```python
from build123d import *

# Parameters (mm, degrees)
SKETCH1_W                    = 152.4
SKETCH1_H                    = 6.35
BOSS_EXTRUDE1_DEPTH          = 126.8095
F_3_4_0_75_DIAMETER_HOLE1_D  = 19.05
CUT_EXTRUDE1_DEPTH           = 199.360106348
FILLET1_R                    = 3.81
FILLET4_R                    = 3.175
F_5_8_0_625_DIAMETER_HOLE1_D = 15.875
F_10_24_TAPPED_HOLE1_D       = 3.7973
F_10_24_TAPPED_HOLE1_DEPTH   = 19.05
F_10_24_TAPPED_HOLE1_TIP     = 1.140824014
F_10_24_TAPPED_HOLE2_D       = 3.7973
F_10_24_TAPPED_HOLE2_DEPTH   = 19.05
F_10_24_TAPPED_HOLE2_TIP     = 1.140824014


with BuildPart() as part:
    # Sketch1 → Boss-Extrude1 (new, symmetric)
    with BuildSketch(Plane.XY):
        with Locations((76.2, 3.175)):
            Rectangle(SKETCH1_W, SKETCH1_H)
    extrude(amount=BOSS_EXTRUDE1_DEPTH, both=True)

    # 3/4 (0.75) Diameter Hole1 (through all)
    with Locations(Plane(origin=(0, 6.35, 0), x_dir=(1, 0, 0), z_dir=(0, 1, 0))):
        with Locations((19.05, 0), (133.35, 0)):
            Hole(F_3_4_0_75_DIAMETER_HOLE1_D / 2)

    # Sketch4 → Cut-Extrude1 (cut, through all)
    with BuildSketch(Plane(origin=(0, 6.35, 0), x_dir=(1, 0, 0), z_dir=(0, 1, 0))):
        with BuildLine():
            Line((37.010512242, -6.35), (64.976021122, -6.35))
            Line((64.976021122, -6.35), (12.7, -93.346011817))
            Line((12.7, -93.346011817), (12.7, -17.960512242))
            ThreePointArc((12.7, -17.960512242), (27.259871939, -17.190128061), (37.010512242, -6.35))
        make_face()
        with BuildLine():
            Line((12.7, 93.346011817), (64.976021122, 6.35))
            Line((64.976021122, 6.35), (37.010512242, 6.35))
            ThreePointArc((37.010512242, 6.35), (27.259871939, 17.190128061), (12.7, 17.960512242))
            Line((12.7, 17.960512242), (12.7, 93.346011817))
        make_face()
        Polygon((137.360297537, 114.1095), (82.55, 22.896029849), (82.55, 114.1095), align=None)
        Polygon((15.039702463, 114.1095), (69.85, 22.896029849), (69.85, 114.1095), align=None)
        with BuildLine():
            Line((139.7, 93.346011817), (87.423978878, 6.35))
            Line((87.423978878, 6.35), (115.389487758, 6.35))
            ThreePointArc((115.389487758, 6.35), (125.140128061, 17.190128061), (139.7, 17.960512242))
            Line((139.7, 17.960512242), (139.7, 93.346011817))
        make_face()
        Polygon((15.039702463, -114.1095), (69.85, -114.1095), (69.85, -22.896029849), align=None)
        with BuildLine():
            Line((139.7, -93.346011817), (139.7, -17.960512242))
            ThreePointArc((139.7, -17.960512242), (125.140128061, -17.190128061), (115.389487758, -6.35))
            Line((115.389487758, -6.35), (87.423978878, -6.35))
            Line((87.423978878, -6.35), (139.7, -93.346011817))
        make_face()
        Polygon((82.55, -22.896029849), (137.360297537, -114.1095), (82.55, -114.1095), align=None)
    extrude(amount=-CUT_EXTRUDE1_DEPTH, mode=Mode.SUBTRACT)

    # Fillet1
    fillet1_edges = [part.edges().sort_by_distance(p)[0] for p in [
        (64.976021122, 3.175, 6.35),
        (12.7, 3.175, 93.346011817),
        (12.7, 3.175, 17.960512242),
        (37.010512242, 3.175, 6.35),
        (139.7, 3.175, -93.346011817),
        (139.7, 3.175, -17.960512242),
        (115.389487758, 3.175, -6.35),
        (87.423978878, 3.175, -6.35),
        (115.389487758, 3.175, 6.35),
        (139.7, 3.175, 17.960512242),
        (139.7, 3.175, 93.346011817),
        (87.423978878, 3.175, 6.35),
        (12.7, 3.175, -17.960512242),
        (12.7, 3.175, -93.346011817),
        (64.976021122, 3.175, -6.35),
        (37.010512242, 3.175, -6.35),
        (15.039702463, 3.175, 114.1095),
        (69.85, 3.175, 22.896029849),
        (69.85, 3.175, 114.1095),
        (137.360297537, 3.175, 114.1095),
        (82.55, 3.175, 114.1095),
        (82.55, 3.175, 22.896029849),
        (82.55, 3.175, -114.1095),
        (137.360297537, 3.175, -114.1095),
        (82.55, 3.175, -22.896029849),
        (15.039702463, 3.175, -114.1095),
        (69.85, 3.175, -114.1095),
        (69.85, 3.175, -22.896029849),
    ]]
    fillet(fillet1_edges, radius=FILLET1_R)

    # Fillet4
    fillet4_edges = [part.edges().sort_by_distance(p)[0] for p in [
        (142.875, 6.35, 0),
        (142.875, 0, 0),
        (28.575, 6.35, 0),
        (28.575, 0, 0),
    ]]
    fillet(fillet4_edges, radius=FILLET4_R - 0.0001)  # a hair under: the kernel refuses the full size

    # 5/8 (0.625) Diameter Hole1 (through all)
    with Locations(Plane(origin=(0, 0, 0), x_dir=(-1, 0, 0), z_dir=(0, -1, 0))):
        with Locations((-76.2, 17.4625), (-76.2, -17.4625)):
            Hole(F_5_8_0_625_DIAMETER_HOLE1_D / 2)

    # #10-24 Tapped Hole1
    with Locations(Plane.XY.offset(126.8095)):
        with Locations((127, 3.175), (25.4, 3.175)):
            Hole(F_10_24_TAPPED_HOLE1_D / 2, depth=F_10_24_TAPPED_HOLE1_DEPTH)
            with Locations((0, 0, -(F_10_24_TAPPED_HOLE1_DEPTH + F_10_24_TAPPED_HOLE1_TIP / 2))):  # 118° drill point
                Cone(0, F_10_24_TAPPED_HOLE1_D / 2, F_10_24_TAPPED_HOLE1_TIP, mode=Mode.SUBTRACT)

    # #10-24 Tapped Hole2
    with Locations(Plane(origin=(0, 0, -126.8095), x_dir=(-1, 0, 0), z_dir=(0, 0, -1))):
        with Locations((-25.4, 3.175), (-127, 3.175)):
            Hole(F_10_24_TAPPED_HOLE2_D / 2, depth=F_10_24_TAPPED_HOLE2_DEPTH)
            with Locations((0, 0, -(F_10_24_TAPPED_HOLE2_DEPTH + F_10_24_TAPPED_HOLE2_TIP / 2))):  # 118° drill point
                Cone(0, F_10_24_TAPPED_HOLE2_D / 2, F_10_24_TAPPED_HOLE2_TIP, mode=Mode.SUBTRACT)


solid = part.part
```
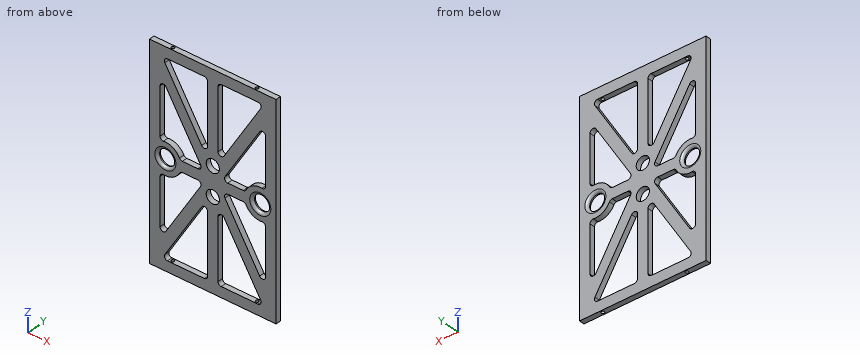
Here's how the part is built. I have some questions about the finished solid (model axes, mm). Coordinates: 2 decimals unless noted, no trailing zeros. Loops run counter-clockwise (first coordinate to the right, second up) from the corner with the lowest first, then second, coordinate; pieces in that order, holes last. Notation, with made-up numbers: M 18,-37 L 24,-37 A20 ccw 24,-21 Z; hole C 78.5,71.25 d4. An arc over 180 degrees is marked long. One line per item, written item: value.
1. Imagine slicing it at C-C (x = 102.5). List the corners of the cut face in (y, z) for me, and give its area (3 significant figures).
Geometry says:
outline: M 0,-126.81 L 6.35,-126.81 L 6.35,-114.11 L 0,-114.11 Z; M 0,-56.1 L 6.35,-56.1 L 6.35,-31.44 L 0,-31.44 Z; M 0,-6.35 L 6.35,-6.35 L 6.35,6.35 L 0,6.35 Z; M 0,31.44 L 6.35,31.44 L 6.35,56.1 L 0,56.1 Z; M 0,114.11 L 6.35,114.11 L 6.35,126.81 L 0,126.81 Z
area: 555 mm2
2. Please list where these lines run through material, in increasing order: probe 1 along Z at (x, y) = (86, 4.5); probe 2 along X at (y, z) = (3.25, 0); probe 3 along Y at (x, z) = (25.4, 117.5).
Geometry says:
probe 1: z = -126.81 to -114.09, -32.84 to 32.84, 114.09 to 126.81
probe 2: x = 0 to 9.52, 28.58 to 123.82, 142.88 to 152.4
probe 3: y = 0 to 1.28, 5.07 to 6.35
3. Imagine slicing it at A-A (x = 76.2). State how many separate pieces and enclosed holes the cut face has, and give its area (3 significant figures).
Geometry says:
separate pieces: 3
enclosed holes: 0
area: 1,410 mm2
4. Will these pins go through, and if not, where does the flat tip stop? pin 1 Ø2.5 at (x, y) = (25.4, 3.175) entering from +Z; pin 2 Ø3 at (x, y) = (25.4, 3.175) entering from +Z; pin 3 Ø2.5 at (x, y) = (127, 3.175) entering from -Z.
Geometry says:
pin 1: stops at z = 98.95
pin 2: stops at z = 99.36
pin 3: stops at z = -98.95
5. Imagine slicing it at D-D (z = -66). List the corners of the cut face in (x, y) for me, and give its area (3 significant figures).
Geometry says:
outline: M 0,0 L 12.7,0 L 12.7,6.35 L 0,6.35 Z; M 29.13,0 L 43.95,0 L 43.95,6.35 L 29.13,6.35 Z; M 69.85,0 L 82.55,0 L 82.55,6.35 L 69.85,6.35 Z; M 108.45,0 L 123.27,0 L 123.27,6.35 L 108.45,6.35 Z; M 139.7,0 L 152.4,0 L 152.4,6.35 L 139.7,6.35 Z
area: 430 mm2
